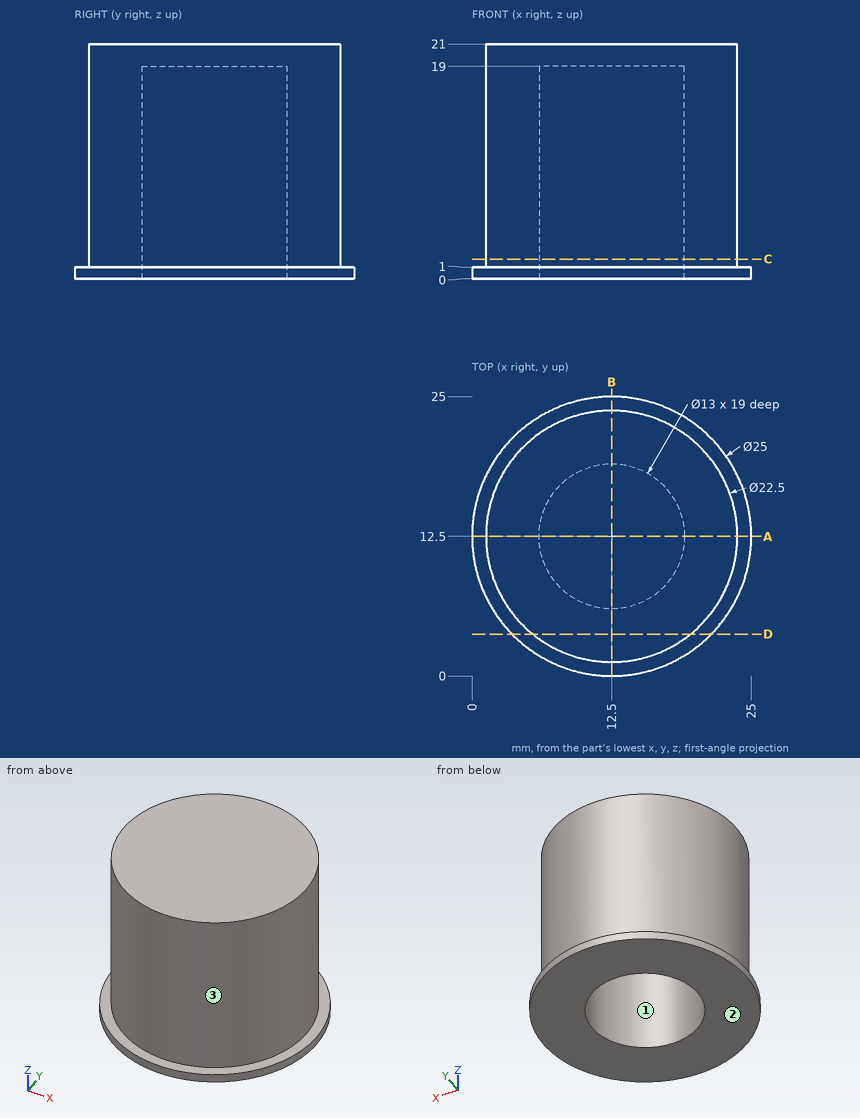
Input: dimensioned drawing with shaded views. Units: mm. Origin: part minimum x, y, z. Round coordinates to 2 decimals unless told otherwise and drop trailing zeros. Loops run counter-clockwise (first coordinate to the right, second up) from the corner with the lowest first, then second, coordinate; pieces in that order, holes last. Notation, with made-up numbers: M 18,36.25 L 61,36.25 A17 cw 61,57.25 Z; hole C 48.5,-7 d6. An arc over 180 degrees is marked long. Answer in a Markdown table with one row per item. Add a question column.
1. Section A-A (y = 12.5). Output: boundary loops of the cut face in (x, z), and give its area (3 significant figures).
2. Section D-D (y = 3.75). Output: boundary loops of the cut face in (x, z), and give its area (3 significant figures).
3. Mould query, pull axis Y, two halves, no side actions, for the marked faces 1, 2 and 3. Classes: released by +Y, released by -Y, zero draft, split by the parting line, or undercut.
4. Contact query for flat-ended pins moving along their axis: pin 1 (10.5 mm diameter, centred on x = 15.5, y = 12.5, fed in from -Z); pin 2 (6 mm diameter, centred on x = 6, z = 8, fed in from +Y); pin 3 (3 mm diameter, centred on x = 10.5, z = 3, fed in from -Y); pin 4 (2 mm diameter, centred on y = 13, z = 9, fed in from +X). Output: stop coordinate, or through.
5. Ray query, probe 1 along Y at (x, z) = (12.5, 7.75); probe 2 along Z at (x, y) = (15.25, 10.75); probe 3 along X at (y, z) = (12, 14.5). Return the intervals inside material, ascending.
6. Section C-C (z = 1.75). Output: boundary loops of the cut face in (x, y), and give its area (3 significant figures).
Values follow:
| question | item | result |
|---|---|---|
| 1 | outline | M 0,0 L 6,0 L 6,19 L 19,19 L 19,0 L 25,0 L 25,1 L 23.75,1 L 23.75,21 L 1.25,21 L 1.25,1 L 0,1 Z |
| 1 | area | 228 mm^2 |
| 2 | outline | M 3.57,0 L 21.43,0 L 21.43,1 L 19.57,1 L 19.57,21 L 5.43,21 L 5.43,1 L 3.57,1 Z |
| 2 | area | 301 mm^2 |
| 3 | face 1 | undercut |
| 3 | face 2 | zero draft |
| 3 | face 3 | split by the parting line |
| 4 | pin 1 | z = 0 |
| 4 | pin 2 | y = 23.19 |
| 4 | pin 3 | y = 1.26 |
| 4 | pin 4 | x = 23.75 |
| 5 | probe 1 | 1.25 to 6, 19 to 23.75 |
| 5 | probe 2 | 19 to 21 |
| 5 | probe 3 | 1.26 to 6.02, 18.98 to 23.74 |
| 6 | outline | C 12.5,12.5 d22.5; hole C 12.5,12.5 d13 |
| 6 | area | 265 mm^2 |
